Model file for the job. Use its own axes, mm. A direction names the side the tool comes from. Coordinates: 2 decimals unless noted, no trailing zeros. Loops run counter-clockwise (first coordinate to the right, second up) from the corner with the lowest first, then second, coordinate; pieces in that order, holes last. Notation, with made-up numbers: M -22,42.5 L 3,42.5 A12 ccw 3,46.5 Z; hole C 84.5,-4 d5. An arc over 180 degrees is marked long. One line per question, with ' | ' between items. Start each with the question number.
```python
from build123d import *

# Parameters (mm, degrees)
BOSS_EXTRU_1_DEPTH                = 57.15
ESQUISSE2_W                       = 25.4
ESQUISSE2_H                       = 47.625
ESQUISSE2_H_2                     = 39.6875
ESQUISSE2_W_2                     = 34.925
ESQUISSE2_H_3                     = 11.1125
ENL_V_MAT_EXTRU_1_DEPTH           = 92.139645599
CHANFREIN1_SIZE                   = 9.525
DIAM_TRE_DU_PER_AGE_5_8_0_625_2_D = 15.875
DIAM_TRE_DU_PER_AGE_1_2_0_5_1_D   = 12.7


with BuildPart() as part:
    # Esquisse1 → Boss.-Extru.1 (new, symmetric)
    with BuildSketch(Plane(origin=(0, 0, 0), x_dir=(0, 0, -1), z_dir=(1, 0, 0))):
        with BuildLine():
            Line((-15.875, 59.683519733), (-15.875, 0))
            Line((-15.875, 0), (15.875, 0))
            Line((15.875, 0), (15.875, 59.683519733))
            ThreePointArc((15.875, 59.683519733), (0, 63.5), (-15.875, 59.683519733))
        make_face()
    extrude(amount=BOSS_EXTRU_1_DEPTH, both=True)

    # Esquisse2 → Enlèv. mat.-Extru.1 (cut, through all)
    with BuildSketch(Plane.XY.offset(15.875)):
        with Locations((44.45, 39.6875)):
            Rectangle(ESQUISSE2_W, ESQUISSE2_H)
        with Locations((-44.45, 39.6875)):
            Rectangle(ESQUISSE2_W, ESQUISSE2_H)
        with Locations((0, 43.65625)):
            Rectangle(ESQUISSE2_W, ESQUISSE2_H_2)
        with Locations((1.5875, 5.55625)):
            Rectangle(ESQUISSE2_W_2, ESQUISSE2_H_3)
    extrude(amount=-ENL_V_MAT_EXTRU_1_DEPTH, mode=Mode.SUBTRACT)

    # Chanfrein1
    chanfrein1_edges = [part.edges().sort_by_distance(p)[0] for p in [
        (-57.15, 7.9375, 15.875),
        (57.15, 7.9375, 15.875),
    ]]
    chamfer(chanfrein1_edges, length=CHANFREIN1_SIZE)

    # Diamètre du perçage 5/8 (0.625)2 (through all)
    with Locations(Plane(origin=(31.75, 0, 0), x_dir=(0, 0, -1), z_dir=(1, 0, 0))):
        with Locations((0, 46.0375)):
            Hole(DIAM_TRE_DU_PER_AGE_5_8_0_625_2_D / 2)

    # Diamètre du perçage 1/2 (0.5)1 (through all)
    with Locations(Plane(origin=(0, 15.875, 0), x_dir=(1, 0, 0), z_dir=(0, 1, 0))):
        with Locations((44.45, 3.175)):
            diam_tre_du_per_age_1_2_0_5_1 = Hole(DIAM_TRE_DU_PER_AGE_1_2_0_5_1_D / 2)

    # Symétrie1: Diamètre du perçage 1/2 (0.5)1 across plane
    add(diam_tre_du_per_age_1_2_0_5_1.mirror(Plane(origin=(0, 0, 0), x_dir=(0, 0, 1), z_dir=(1, 0, 0))), mode=Mode.SUBTRACT)


solid = part.part
```
(1) Band-saw the part on D-D on z = 1.5. Give the number of separate pieces and of enclosed holes in the cut face, then the cut area to 3 significant figures.
(2) Drill centre lines: line 1 (Z direction, x = 44.45, y = 10.25) (3 decimals); line 2 (X direction, y = 31, z = 10.5); line 3 (X direction, y = 19, z = -13). Where is each one in solid material? Low to high. Write a range as [from, to].
(3) Band-saw the part on B-B on y = 33. Write the cut outline in (x, z) (3 decimals).
(4) 3-axis set-ups, long thin cutter, end or side, ignore diameter. For faces 4 (the face through (44, 15.875, 4)), 5 (the face through (-31.75, 34, 0)), 6 (the face through (1, 11.112, 0)): which of +Z, -Z, +X, -X, +Y, -Y reach the whole face in a straight line?
(5) Two-plate mould, pull along Z, no slides. Class faces 1 (the face through (-22.1, 63.5, -0.2)), 2 (the face through (-38.4, 7.8, -5.1)), 3 (the face through (-57.15, 8, -5)): pulls with the +Z half, pulls with the -Z half, needs draft (parallel to the pull), parting line crosses it, or undercut.
(6) Band-saw the part on C-C on y = 40.5. Write the cut outline in (x, z) (3 decimals), then the cut area to 3 significant figures.
(7) Band-saw the part on A-A on x = 44.45. Write the cut outline in (y, z) (3 decimals).
(8) Pin check, flat tips, straight feed: P1, Ø1, axis at y = 26, z = -0.5, coming from the +X side; P2, Ø6, axis at y = 45.5, z = 12, coming from the -X side; P3, Ø12.5, axis at x = 45, z = 1.5, coming from the +Y side (3 decimals); P4, Ø12, axis at x = -13.5, z = -4, coming from the -Y side. Stop position of each tip, or through.
Computed values:
1) separate pieces: 5 | enclosed holes: 0 | area: 2,570 mm^2
2) line 1: [-15.875, -9.525], [3.175, 15.875] | line 2: [-31.75, -12.7], [12.7, 31.75] | line 3: [-31.75, 31.75]
3) outline: M -31.75,-15.875 L -12.7,-15.875 L -12.7,15.875 L -31.75,15.875 Z; M 12.7,-15.875 L 31.75,-15.875 L 31.75,15.875 L 12.7,15.875 Z
4) face 4: +Z, -Z, +X, +Y | face 5: +Z, -Z, -X, +Y | face 6: +Z, -Z, -Y
5) face 1: parting line crosses it | face 2: undercut | face 3: needs draft
6) outline: M -31.75,-15.875 L -12.7,-15.875 L -12.7,-5.687 L -31.75,-5.687 Z; M -31.75,5.687 L -12.7,5.687 L -12.7,15.875 L -31.75,15.875 Z; M 12.7,-15.875 L 31.75,-15.875 L 31.75,-5.687 L 12.7,-5.687 Z; M 12.7,5.687 L 31.75,5.687 L 31.75,15.875 L 12.7,15.875 Z | area: 776 mm^2
7) outline: M 0,-15.875 L 15.875,-15.875 L 15.875,-9.525 L 0,-9.525 Z; M 0,3.175 L 15.875,3.175 L 15.875,15.875 L 0,15.875 Z
8) P1: x = 31.75 | P2: x = -31.75 | P3: y = 15.875 | P4: y = 0
